from build123d import *

# Parameters (mm, degrees)
BOSS_EXTRUDE1_DEPTH     = 33.8
CUT_EXTRUDE1_DEPTH      = 40
CUT_EXTRUDE1_DEPTH_BACK = 40
SKETCH13_R              = 4
BOSS_EXTRUDE2_DEPTH     = 1.3
SKETCH14_R              = 4
BOSS_EXTRUDE3_DEPTH     = 1.3
SKETCH15_W              = 2.2
SKETCH15_H              = 35.1
SKETCH17_W              = 2.2
SKETCH17_H              = 35.1
SKETCH18_W              = 2.5
SKETCH18_H              = 5
BOSS_EXTRUDE4_DEPTH     = 1.5
SKETCH19_W              = 2
SKETCH19_H              = 5
BOSS_EXTRUDE5_DEPTH     = 1.5


with BuildPart() as part:
    # Sketch1 → Boss-Extrude1 (new body)
    with BuildSketch(Plane(origin=(0, 1.3, 0), x_dir=(1, 0, 0), z_dir=(0, 1, 0))):
        with BuildLine():
            Line((-12.75, -53.65), (38.4, -53.65))
            Line((38.4, -53.65), (38.4, -22.654162541))
            ThreePointArc((38.4, -22.654162541), (38.338748223, -22.414370972), (38.170000014, -22.233330042))
            ThreePointArc((38.170000014, -22.233330042), (37.258228535, -20.731235846), (37.883912522, -19.089245057))
            Line((37.883912522, -19.089245057), (38.97947873, -18.064679449))
            ThreePointArc((38.97947873, -18.064679449), (39.538283152, -16.544955205), (38.649999929, -15.191154232))
            ThreePointArc((38.649999929, -15.191154232), (38.466987278, -15.008141536), (38.4, -14.758141571))
            Line((38.4, -14.758141571), (38.4, 53.65))
            Line((38.4, 53.65), (-12.75, 53.65))
            Line((-12.75, 53.65), (-12.75, -53.65))
        make_face()
    extrude(amount=BOSS_EXTRUDE1_DEPTH)

    # Sketch2 → Cut-Extrude1 (cut, two sides)
    with BuildSketch(Plane(origin=(0, 0, 0), x_dir=(0, 0, -1), z_dir=(1, 0, 0))) as cut_extrude1_sk:
        Polygon((-26, 2.9), (-26, -8.174443219), (14, -7.963716906), (14, 2.543524479), (16.45, 3.2), (16.45, 4.4), (-19.05, 4.4), (-19.05, 2.9), align=None)
    extrude(amount=CUT_EXTRUDE1_DEPTH, mode=Mode.SUBTRACT)
    extrude(cut_extrude1_sk.sketch, amount=-CUT_EXTRUDE1_DEPTH_BACK, mode=Mode.SUBTRACT)

    # Sketch3 → Cut-Revolve1 (revolve, cut)
    with BuildSketch(Plane(origin=(28.5, 0, 0), x_dir=(0, 0, -1), z_dir=(1, 0, 0))):
        Polygon((-53.65, 9.8), (-53.65, 16.3785), (-52.794, 15.5225), (-35.65, 15.5225), (-35.65, 9.8), align=None)
    revolve(axis=Axis((28.5, 9.8, 35.65), (0, 0, 1)), mode=Mode.SUBTRACT)

    # Sketch4 → Cut-Revolve2 (revolve, cut)
    with BuildSketch(Plane(origin=(25.5, 0, 0), x_dir=(0, 0, -1), z_dir=(1, 0, 0))):
        Polygon((-53.65, 23.9), (-53.65, 27.65), (-52.86, 26.86), (-44.65, 26.86), (-44.65, 23.9), align=None)
    revolve(axis=Axis((25.5, 23.9, 44.65), (0, 0, 1)), mode=Mode.SUBTRACT)

    # Sketch5 → Cut-Revolve3 (revolve, cut)
    with BuildSketch(Plane(origin=(1.25, 0, 0), x_dir=(0, 0, -1), z_dir=(1, 0, 0))):
        Polygon((47.65, 35.1), (49.15, 35.1), (48.8795, 34.8295), (48.8795, 30.1), (47.65, 30.1), align=None)
    revolve(axis=Axis((1.25, 30.1, -47.65), (0, 1, 0)), mode=Mode.SUBTRACT)

    # Sketch6 → Cut-Revolve4 (revolve, cut)
    with BuildSketch(Plane(origin=(1.25, 0, 0), x_dir=(0, 0, -1), z_dir=(1, 0, 0))):
        Polygon((-47.65, 35.1), (-46.15, 35.1), (-46.4205, 34.8295), (-46.4205, 30.1), (-47.65, 30.1), align=None)
    revolve(axis=Axis((1.25, 30.1, 47.65), (0, 1, 0)), mode=Mode.SUBTRACT)

    # Sketch7 → Cut-Revolve5 (revolve, cut)
    with BuildSketch(Plane(origin=(23.5, 0, 0), x_dir=(0, 0, -1), z_dir=(1, 0, 0))):
        Polygon((-38.05, 35.1), (-36.55, 35.1), (-36.8205, 34.8295), (-36.8205, 30.1), (-38.05, 30.1), align=None)
    revolve(axis=Axis((23.5, 30.1, 38.05), (0, 1, 0)), mode=Mode.SUBTRACT)

    # Sketch8 → Cut-Revolve6 (revolve, cut)
    with BuildSketch(Plane(origin=(23.5, 0, 0), x_dir=(0, 0, -1), z_dir=(1, 0, 0))):
        Polygon((0.75, 35.1), (2.25, 35.1), (1.9795, 34.8295), (1.9795, 30.1), (0.75, 30.1), align=None)
    revolve(axis=Axis((23.5, 30.1, -0.75), (0, 1, 0)), mode=Mode.SUBTRACT)

    # Sketch9 → Cut-Revolve7 (revolve, cut)
    with BuildSketch(Plane(origin=(23.5, 0, 0), x_dir=(0, 0, -1), z_dir=(1, 0, 0))):
        Polygon((50.75, 35.1), (52.25, 35.1), (51.9795, 34.8295), (51.9795, 30.1), (50.75, 30.1), align=None)
    revolve(axis=Axis((23.5, 30.1, -50.75), (0, 1, 0)), mode=Mode.SUBTRACT)

    # Sketch10 → Cut-Revolve8 (revolve, cut)
    with BuildSketch(Plane(origin=(35.3, 0, 0), x_dir=(0, 0, -1), z_dir=(1, 0, 0))):
        Polygon((-38.05, 35.1), (-36.55, 35.1), (-36.8205, 34.8295), (-36.8205, 30.1), (-38.05, 30.1), align=None)
    revolve(axis=Axis((35.3, 30.1, 38.05), (0, 1, 0)), mode=Mode.SUBTRACT)

    # Sketch11 → Cut-Revolve9 (revolve, cut)
    with BuildSketch(Plane(origin=(35.3, 0, 0), x_dir=(0, 0, -1), z_dir=(1, 0, 0))):
        Polygon((0.75, 35.1), (2.25, 35.1), (1.9795, 34.8295), (1.9795, 30.1), (0.75, 30.1), align=None)
    revolve(axis=Axis((35.3, 30.1, -0.75), (0, 1, 0)), mode=Mode.SUBTRACT)

    # Sketch12 → Cut-Revolve10 (revolve, cut)
    with BuildSketch(Plane(origin=(35.3, 0, 0), x_dir=(0, 0, -1), z_dir=(1, 0, 0))):
        Polygon((50.75, 35.1), (52.25, 35.1), (51.9795, 34.8295), (51.9795, 30.1), (50.75, 30.1), align=None)
    revolve(axis=Axis((35.3, 30.1, -50.75), (0, 1, 0)), mode=Mode.SUBTRACT)

    # Sketch13 → Boss-Extrude2 (add)
    with BuildSketch(Plane(origin=(0, 1.3, 0), x_dir=(-1, 0, 0), z_dir=(0, -1, 0))):
        with Locations((-17.65, -46.15)):
            Circle(SKETCH13_R)
    extrude(amount=BOSS_EXTRUDE2_DEPTH)

    # Sketch14 → Boss-Extrude3 (add)
    with BuildSketch(Plane(origin=(0, 1.3, 0), x_dir=(-1, 0, 0), z_dir=(0, -1, 0))):
        with Locations((-17.65, 20.15)):
            Circle(SKETCH14_R)
    extrude(amount=BOSS_EXTRUDE3_DEPTH)

    # Sketch15 → Cut-Revolve11 (revolve, cut)
    with BuildSketch(Plane(origin=(17.25, 0, 0), x_dir=(0, 0, -1), z_dir=(1, 0, 0))):
        with Locations((-45.05, 17.55)):
            Rectangle(SKETCH15_W, SKETCH15_H)
    revolve(axis=Axis((17.25, 0, 46.15), (0, 1, 0)), mode=Mode.SUBTRACT)

    # Sketch16 → Cut-Revolve12 (revolve, cut)
    with BuildSketch(Plane(origin=(17.25, 0, 0), x_dir=(0, 0, -1), z_dir=(1, 0, 0))):
        Polygon((-23.05, 35.1), (-18.55, 35.1), (-18.55, 10.1), (-20.85, 10.1), (-20.85, 0), (-23.05, 0), align=None)
    revolve(axis=Axis((17.25, 0, 23.05), (0, 1, 0)), mode=Mode.SUBTRACT)

    # Sketch17 → Cut-Revolve13 (revolve, cut)
    with BuildSketch(Plane(origin=(17.25, 0, 0), x_dir=(0, 0, -1), z_dir=(1, 0, 0))):
        with Locations((21.25, 17.55)):
            Rectangle(SKETCH17_W, SKETCH17_H)
    revolve(axis=Axis((17.25, 0, -20.15), (0, 1, 0)), mode=Mode.SUBTRACT)

    # Sketch18 → Boss-Extrude4 (add)
    with BuildSketch(Plane(origin=(0, 0, 0), x_dir=(1, 0, 0), z_dir=(0, 1, 0))):
        with Locations((37.15, 38.55)):
            Rectangle(SKETCH18_W, SKETCH18_H)
    extrude(amount=BOSS_EXTRUDE4_DEPTH)

    # Sketch19 → Boss-Extrude5 (add)
    with BuildSketch(Plane(origin=(0, 0, 0), x_dir=(1, 0, 0), z_dir=(0, 1, 0))):
        with Locations((-3.65, 38.55)):
            Rectangle(SKETCH19_W, SKETCH19_H)
    extrude(amount=BOSS_EXTRUDE5_DEPTH)


solid = part.part
Work out the finished part from the listing and answer in its coordinate system (mm). A direction names the side the tool comes from. Give positions to 0.01 mm unless a question says otherwise; leave off trailing zeros. Loops run counter-clockwise (first coordinate to the right, second up) from the corner with the lowest first, then second, coordinate; pieces in that order, holes last. Notation, with made-up numbers: (31.25, 40.5) - (67.25, 40.5) arc R20 cw to (67.25, 70.5) - close; hole circle Ø10 at (33, 66). An arc over 180 degrees is marked (long way). Answer in a Markdown table with one row per item. Add a question column.
Q1. Determine the mould class of faces 1 (the flat face through (13.183, 2.867, -15.208)), 2 (the flat face through (37, 0, -39)), 3 (the flat face through (25, 24, 44.65)) for opening direction Z: released by +Z, released by -Z, zero draft, split by the parting line, or undercut.
Q2. The part is cut by section D-D (z = 3). Determine the outline of the cut face in (x, y).
Q3. A tool of negligible diameter and unlimited length cuts with its end or side. For faces 4 (the flat face through (19.5, 0, 47)), 5 (the flat face through (38.4, 17, -19)), 6 (the cylindrical face through (36.5, 32.43, 38.32)), from which of +Z, -Z, +X, -X, +Y, -Y can it reach the whole face along a straight path? Write none if from no direction.
Q4. The part is cut by section B-B (x = 1.25). Determine the outline of the cut face in (y, z).
Q5. Each of these flat-tipped pins is pushed along its axis until it touches: P1, Ø2.5, axis at x = 17.25, z = 46.15, coming from the +Y side; P2, Ø6, axis at x = 27, y = 27, coming from the +Z side; P3, Ø0.7, axis at x = 1.5, z = 47.5, coming from the +Y side; P4, Ø5.5, axis at x = 7, z = 24, coming from the -Y side. Where does it stop, or does it pass through?
Q6. The part is cut by section A-A (y = 23.9). Determine the outline of the cut face in (x, z), and give its area (3 significant figures).
Q7. Consider line 1 along X through (y, z) = (33, 38); line 2 along Z through (x, y) = (17.25, 21.5); line 3 along X through (y, z) = (8, 23.05). Determine where each line is inside the solid, lowest interval first.
Solution:
| question | item | result |
|---|---|---|
| 1 | face 1 | undercut |
| 1 | face 2 | zero draft |
| 1 | face 3 | released by +Z |
| 2 | outline | (-12.75, 4.4) - (38.4, 4.4) - (38.4, 35.1) - (-12.75, 35.1) - close |
| 3 | face 4 | +Z, -Z, +X, -X, -Y |
| 3 | face 5 | -Z, +X, +Y, -Y |
| 3 | face 6 | +Y |
| 4 | outline | (1.3, -53.65) - (35.1, -53.65) - (35.1, -49.15) - (34.83, -48.88) - (30.1, -48.88) - (30.1, -46.42) - (34.83, -46.42) - (35.1, -46.15) - (35.1, 46.15) - (34.83, 46.42) - (30.1, 46.42) - (30.1, 48.88) - (34.83, 48.88) - (35.1, 49.15) - (35.1, 53.65) - (1.3, 53.65) - (1.3, 26) - (2.9, 26) - (2.9, 19.05) - (4.4, 19.05) - (4.4, -16.45) - (3.2, -16.45) - (2.54, -14) - (1.3, -14) - close |
| 5 | P1 | passes through |
| 5 | P2 | stops at z = 53.65 |
| 5 | P3 | stops at y = 30.1 |
| 5 | P4 | stops at y = 1.3 |
| 6 | outline | (-12.75, -53.65) - (38.4, -53.65) - (38.4, 14.76) arc R0.5 cw to (38.65, 15.19) arc R1.8 ccw to (38.98, 18.06) - (37.88, 19.09) arc R2 cw to (38.17, 22.23) arc R0.5 ccw to (38.4, 22.65) - (38.4, 53.65) - (29.25, 53.65) - (28.46, 52.86) - (28.46, 44.65) - (22.54, 44.65) - (22.54, 52.86) - (21.75, 53.65) - (-12.75, 53.65) - close; hole circle Ø9 at (17.25, 23.05); hole circle Ø4.4 at (17.25, -20.15); hole circle Ø4.4 at (17.25, 46.15) |
| 6 | area | 5,340 mm² |
| 7 | line 1 | x = -12.75 to 22.27, 24.73 to 34.07, 36.53 to 38.4 |
| 7 | line 2 | z = -53.65 to -22.35, -17.95 to 18.55, 27.55 to 43.95, 48.35 to 53.65 |
| 7 | line 3 | x = -12.75 to 15.05, 19.45 to 38.4 |
